```python
from build123d import *

# Parameters (mm, degrees)
SKETCH1_W              = 20
SKETCH1_H              = 12
BOSS_EXTRUDE1_DEPTH    = 22
M6X1_0_TAPPED_HOLE1_D  = 5
SKETCH7_W              = 2
SKETCH7_H              = 2
CUT_EXTRUDE2_DEPTH     = 46.519226707
M10X1_5_TAPPED_HOLE1_D = 8.5


with BuildPart() as part:
    # Sketch1 → Boss-Extrude1 (new, symmetric)
    with BuildSketch(Plane.XY):
        Rectangle(SKETCH1_W, SKETCH1_H)
    extrude(amount=BOSS_EXTRUDE1_DEPTH, both=True)

    # M6x1.0 Tapped Hole1 (through all)
    with Locations(Plane(origin=(0, 6, 0), x_dir=(1, 0, 0), z_dir=(0, 1, 0))):
        with Locations((0, -15), (0, 0), (0, 15)):
            Hole(M6X1_0_TAPPED_HOLE1_D / 2)

    # Sketch7 → Cut-Extrude2 (cut, through all)
    with BuildSketch(Plane(origin=(0, 0, -22), x_dir=(-1, 0, 0), z_dir=(0, 0, -1))):
        with Locations((0, 5)):
            Rectangle(SKETCH7_W, SKETCH7_H)
    extrude(amount=-CUT_EXTRUDE2_DEPTH, mode=Mode.SUBTRACT)

    # M10x1.5 Tapped Hole1 (through all)
    with Locations(Plane(origin=(0, 6, 0), x_dir=(1, 0, 0), z_dir=(0, 1, 0))):
        with Locations((0, 15)):
            Hole(M10X1_5_TAPPED_HOLE1_D / 2)


solid = part.part
```
Check sheet for the modelled part. Datum: model origin and axes. Units: mm. A direction names the side the tool comes from. Round coordinates to 2 decimals unless told otherwise and drop trailing zeros. Order: outer loops, then holes, each group sorted by start corner. A loop starts at its lowest first (then second) coordinate and runs counter-clockwise, first axis right, second up. Notation, with made-up numbers: (9, 75.5) - (59, 75.5) arc R31 ccw to (59, 113.5) - close; hole circle Ø4 at (4, -15.5). An arc over 180 degrees is marked (long way). Answer as CSV lines item,"result". Start each with the question number.
1) Depth check by flat-ended pin: pin 1 (4 mm diameter, centred on x = 0, z = 15, fed in from +Y); pin 2 (1.5 mm diameter, centred on x = -1, z = 2, fed in from +Y); pin 3 (0.6 mm diameter, centred on x = -0.5, z = 6.5, fed in from +Y). Enter the tip coordinate at first touch or a pass-through.
2) Section check A-A (z = 15). Record the cut outline in (x, y), then the cut area to 3 significant figures.
3) Tool access check on faces 1 (the face through (1, 5, -7)), 2 (the face through (5, 6, 0)). Record the directions out of +Z, -Z, +X, -X, +Y, -Y that give a thin tool (end or side, any length) a straight path to the whole face; none if there is none.
4) Section check D-D (z = -9). Record the cut outline in (x, y).
5) Section check B-B (x = 0). Record the cut outline in (y, z).
6) Draft check along Z on faces 3 (the face through (0, 0, 22)), 4 (the face through (-3.926, -0.084, -13.372)), 5 (the face through (-1, 5, -7)), 6 (the face through (-2.31, -0.08, 15.96)). Enter one of: +Z half, -Z half, draft (parallel to the pull), parting line (faces both ways), or undercut.
7) Scan lines: probe 1 along Z at (x, y) = (0, 2.75); probe 2 along X at (y, z) = (-3.5, 15); probe 3 along Z at (x, y) = (-1.25, -1.25). Record each from-to range of solid material in increasing order.
8) Section check C-C (y = 1). Record the cut outline in (x, z).
Determined:
1,pin 1,"through"
1,pin 2,"y = 6"
1,pin 3,"y = 4"
2,outline,"(-10, -6) - (-2.5, -6) - (-2.5, 6) - (-10, 6) - close; (2.5, -6) - (10, -6) - (10, 6) - (2.5, 6) - close"
2,area,"180 mm^2"
3,face 1,"+Z, -Z, +Y"
3,face 2,"+Z, -Z, +X, -X, +Y"
4,outline,"(-10, -6) - (10, -6) - (10, 6) - (1, 6) - (1, 4) - (-1, 4) - (-1, 6) - (-10, 6) - close"
5,outline,"(-6, -22) - (4, -22) - (4, -19.25) - (-6, -19.25) - close; (-6, -10.75) - (4, -10.75) - (4, -2.5) - (-6, -2.5) - close; (-6, 2.5) - (4, 2.5) - (4, 12.5) - (-6, 12.5) - close; (-6, 17.5) - (4, 17.5) - (4, 22) - (-6, 22) - close"
6,face 3,"+Z half"
6,face 4,"undercut"
6,face 5,"draft"
6,face 6,"undercut"
7,probe 1,"-22 to -19.25, -10.75 to -2.5, 2.5 to 12.5, 17.5 to 22"
7,probe 2,"-10 to -2.5, 2.5 to 10"
7,probe 3,"-22 to -19.06, -10.94 to -2.17, 2.17 to 12.83, 17.17 to 22"
8,outline,"(-10, -22) - (10, -22) - (10, 22) - (-10, 22) - close; hole circle Ø8.5 at (0, -15); hole circle Ø5 at (0, 0); hole circle Ø5 at (0, 15)"
